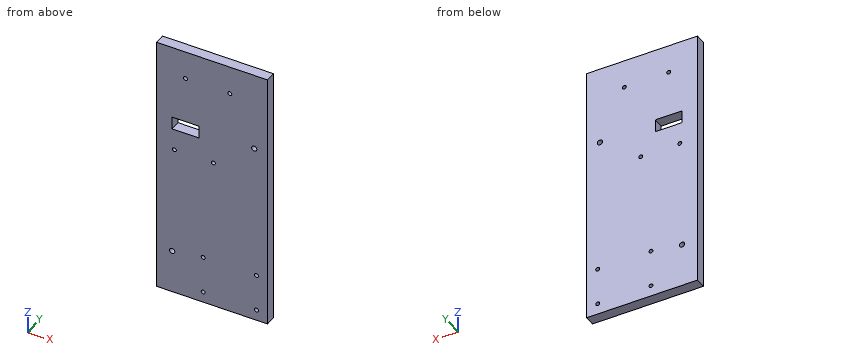
from build123d import *

# Parameters (mm, degrees)
SKETCH1_W             = 63.5
SKETCH1_H             = 152.4
BOSS_EXTRUDE1_DEPTH   = 5.9436
SKETCH4_W             = 15.24
SKETCH4_H             = 7.366
CUT_EXTRUDE3_DEPTH    = 166.206950159
F_4_40_TAPPED_HOLE1_D = 2.2606
F_4_40_TAPPED_HOLE2_D = 2.2606
F_4_40_TAPPED_HOLE3_D = 2.2606
SKETCH13_R            = 1.524
CUT_EXTRUDE5_DEPTH    = 166.206950159


with BuildPart() as part:
    # Sketch1 → Boss-Extrude1 (new body)
    with BuildSketch(Plane(origin=(0, 0, 0), x_dir=(1, 0, 0), z_dir=(0, 1, 0))):
        with Locations((31.75, 76.2)):
            Rectangle(SKETCH1_W, SKETCH1_H)
    extrude(amount=BOSS_EXTRUDE1_DEPTH)

    # Sketch4 → Cut-Extrude3 (cut, through all)
    with BuildSketch(Plane(origin=(0, 5.9436, 0), x_dir=(1, 0, 0), z_dir=(0, 1, 0))):
        with Locations((16.51, 47.117)):
            Rectangle(SKETCH4_W, SKETCH4_H)
    extrude(amount=-CUT_EXTRUDE3_DEPTH, mode=Mode.SUBTRACT)

    # #4-40 Tapped Hole1 (through all)
    with Locations(Plane(origin=(0, 5.9436, 0), x_dir=(1, 0, 0), z_dir=(0, 1, 0))):
        with Locations((57.15, 146.05), (57.15, 124.46), (26.67, 124.46), (26.67, 146.05)):
            Hole(F_4_40_TAPPED_HOLE1_D / 2)

    # #4-40 Tapped Hole2 (through all)
    with Locations(Plane(origin=(0, 5.9436, 0), x_dir=(1, 0, 0), z_dir=(0, 1, 0))):
        with Locations((32.512, 63.3222), (10.16, 63.3222)):
            Hole(F_4_40_TAPPED_HOLE2_D / 2)

    # #4-40 Tapped Hole3 (through all)
    with Locations(Plane(origin=(0, 5.9436, 0), x_dir=(1, 0, 0), z_dir=(0, 1, 0))):
        with Locations((41.91, 16.51), (16.51, 16.51)):
            Hole(F_4_40_TAPPED_HOLE3_D / 2)

    # Sketch13 → Cut-Extrude5 (cut, through all)
    with BuildSketch(Plane(origin=(0, 5.9436, 0), x_dir=(1, 0, 0), z_dir=(0, 1, 0))):
        with Locations(Location((8.89, 127, 0), (0, 0, 270))):
            Circle(SKETCH13_R)
        with Locations(Location((55.88, 45.72, 0), (0, 0, 270))):
            Circle(SKETCH13_R)
    extrude(amount=-CUT_EXTRUDE5_DEPTH, mode=Mode.SUBTRACT)


solid = part.part
The model under review builds one solid part; all positions refer to its coordinate system, in mm. Round coordinates to 2 decimals unless told otherwise and drop trailing zeros. Loops run counter-clockwise (first coordinate to the right, second up) from the corner with the lowest first, then second, coordinate; pieces in that order, holes last. Notation, with made-up numbers: M 11,11 L 37,11 A23 cw 37,35 Z; hole C 24.5,-32 d5. An arc over 180 degrees is marked long. Answer as CSV lines item,"result". Start each with the question number.
Item 1: Wall thickness on line 1 (X direction, y = 2.8, z = -146.05); line 2 (X direction, y = 4.65, z = -16.51); line 3 (Z direction, x = 57.15, y = 1.8): over which ranges is each line inside the solid? List them lowest first. Write a range as [from, to].
Item 2: Consider section B-B (y = 3.95). State how many separate pieces and enclosed holes the cut face has, then the cut area to 3 significant figures.
Item 3: Consider section A-A (z = -127). Write out the cut boundary in (x, y), then the cut area to 3 significant figures.
Answer:
1,line 1,"x = [0, 25.54], [27.8, 56.02], [58.28, 63.5]"
1,line 2,"x = [0, 15.38], [17.64, 40.78], [43.04, 63.5]"
1,line 3,"z = [-152.4, -147.18], [-144.92, -125.59], [-123.33, -46.56], [-44.88, 0]"
2,separate pieces,"1"
2,enclosed holes,"11"
2,area,"9,520 mm^2"
3,outline,"M 0,0 L 7.37,0 L 7.37,5.94 L 0,5.94 Z; M 10.41,0 L 63.5,0 L 63.5,5.94 L 10.41,5.94 Z"
3,area,"359 mm^2"
